from build123d import *

# Parameters (mm, degrees)
SKETCH1_W           = 50
SKETCH1_H           = 50
SKETCH1_R           = 8
BOSS_EXTRUDE1_DEPTH = 1.5
SKETCH4_R           = 1.5
BOSS_EXTRUDE2_DEPTH = 2
BOSS_EXTRUDE3_START = -1.5
SKETCH5_R           = 2.6
SKETCH5_R_2         = 8
BOSS_EXTRUDE3_DEPTH = 1.5
FILLET1_R           = 5
SKETCH6_R           = 5
SKETCH6_R_2         = 2.6
BOSS_EXTRUDE4_DEPTH = 10


with BuildPart() as part:
    # Sketch1 → Boss-Extrude1 (new body)
    with BuildSketch(Plane(origin=(0, 0, 0), x_dir=(1, 0, 0), z_dir=(0, 1, 0))):
        Rectangle(SKETCH1_W, SKETCH1_H)
        with Locations(Location((0, 0, 0), (0, 0, 270))):
            Circle(SKETCH1_R, mode=Mode.SUBTRACT)
    extrude(amount=BOSS_EXTRUDE1_DEPTH)

    # Sketch4 → Boss-Extrude2 (add)
    with BuildSketch(Plane(origin=(0, 1.5, 0), x_dir=(1, 0, 0), z_dir=(0, 1, 0))):
        with Locations(Location((-23, 23, 0), (0, 0, 90))):
            Circle(SKETCH4_R)
        with Locations(Location((-17, 17, 0), (0, 0, 90))):
            Circle(SKETCH4_R)
        with Locations(Location((17, 17, 0), (0, 0, 90))):
            Circle(SKETCH4_R)
        with Locations(Location((23, 23, 0), (0, 0, 90))):
            Circle(SKETCH4_R)
        with Locations(Location((-17, -17, 0), (0, 0, 90))):
            Circle(SKETCH4_R)
        with Locations(Location((-23, -23, 0), (0, 0, 90))):
            Circle(SKETCH4_R)
        with Locations(Location((17, -17, 0), (0, 0, 90))):
            Circle(SKETCH4_R)
        with Locations(Location((23, -23, 0), (0, 0, 90))):
            Circle(SKETCH4_R)
    extrude(amount=BOSS_EXTRUDE2_DEPTH)

    # Sketch5 → Boss-Extrude3 (add)
    with BuildSketch(Plane(origin=(0, 1.5, 0), x_dir=(1, 0, 0), z_dir=(0, 1, 0)).offset(BOSS_EXTRUDE3_START)):
        Polygon((-42.426406871, -35.355339059), (-25, -17.928932188), (-25, 17.928932188), (-42.426406871, 35.355339059), (-45.961940777, 38.890872965), (-38.890872965, 45.961940777), (-35.355339059, 42.426406871), (-17.928932188, 25), (17.928932188, 25), (35.355339059, 42.426406871), (38.890872965, 45.961940777), (45.961940777, 38.890872965), (42.426406871, 35.355339059), (25, 17.928932188), (25, -17.928932188), (42.426406871, -35.355339059), (45.961940777, -38.890872965), (38.890872965, -45.961940777), (35.355339059, -42.426406871), (17.928932188, -25), (-17.928932188, -25), (-35.355339059, -42.426406871), (-38.890872965, -45.961940777), (-45.961940777, -38.890872965), align=None)
        with Locations(Location((-38.890872965, -38.890872965, 0), (0, 0, 270))):
            Circle(SKETCH5_R, mode=Mode.SUBTRACT)
        with Locations(Location((38.890872965, 38.890872965, 0), (0, 0, 270))):
            Circle(SKETCH5_R, mode=Mode.SUBTRACT)
        with Locations(Location((38.890872965, -38.890872965, 0), (0, 0, 90))):
            Circle(SKETCH5_R, mode=Mode.SUBTRACT)
        with Locations(Location((-38.890872965, 38.890872965, 0), (0, 0, 90))):
            Circle(SKETCH5_R, mode=Mode.SUBTRACT)
        with Locations(Location((0, 0, 0), (0, 0, 270))):
            Circle(SKETCH5_R_2, mode=Mode.SUBTRACT)
    extrude(amount=BOSS_EXTRUDE3_DEPTH)

    # Fillet1
    fillet1_edges = [part.edges().sort_by_distance(p)[0] for p in [
        (17.928932188, 0.75, 25),
        (38.890872965, 0.75, 45.961940777),
        (45.961940777, 0.75, 38.890872965),
        (25, 0.75, 17.928932188),
        (25, 0.75, -17.928932188),
        (45.961940777, 0.75, -38.890872965),
        (38.890872965, 0.75, -45.961940777),
        (17.928932188, 0.75, -25),
        (-17.928932188, 0.75, -25),
        (-38.890872965, 0.75, -45.961940777),
        (-45.961940777, 0.75, -38.890872965),
        (-25, 0.75, -17.928932188),
        (-25, 0.75, 17.928932188),
        (-45.961940777, 0.75, 38.890872965),
        (-38.890872965, 0.75, 45.961940777),
        (-17.928932188, 0.75, 25),
    ]]
    fillet(fillet1_edges, radius=FILLET1_R - 0.0001)  # a hair under: the kernel refuses the full size

    # Sketch6 → Boss-Extrude4 (add)
    # profile 1 of 4: a face of its own
    with BuildSketch(Plane(origin=(0, 1.5, 0), x_dir=(1, 0, 0), z_dir=(0, 1, 0))):
        with Locations(Location((-38.890872965, -38.890872965, 0), (0, 0, 270))):
            Circle(SKETCH6_R)
        with Locations(Location((-38.890872965, -38.890872965, 0), (0, 0, 270))):
            Circle(SKETCH6_R_2, mode=Mode.SUBTRACT)
    # profile 2 of 4: a face of its own
    with BuildSketch(Plane(origin=(0, 1.5, 0), x_dir=(1, 0, 0), z_dir=(0, 1, 0))):
        with Locations(Location((-38.890872965, 38.890872965, 0), (0, 0, 270))):
            Circle(SKETCH6_R)
        with Locations(Location((-38.890872965, 38.890872965, 0), (0, 0, 270))):
            Circle(SKETCH6_R_2, mode=Mode.SUBTRACT)
    # profile 3 of 4: a face of its own
    with BuildSketch(Plane(origin=(0, 1.5, 0), x_dir=(1, 0, 0), z_dir=(0, 1, 0))):
        with Locations(Location((38.890872965, 38.890872965, 0), (0, 0, 270))):
            Circle(SKETCH6_R)
        with Locations(Location((38.890872965, 38.890872965, 0), (0, 0, 270))):
            Circle(SKETCH6_R_2, mode=Mode.SUBTRACT)
    # profile 4 of 4: a face of its own
    with BuildSketch(Plane(origin=(0, 1.5, 0), x_dir=(1, 0, 0), z_dir=(0, 1, 0))):
        with Locations(Location((38.890872965, -38.890872965, 0), (0, 0, 270))):
            Circle(SKETCH6_R)
        with Locations(Location((38.890872965, -38.890872965, 0), (0, 0, 270))):
            Circle(SKETCH6_R_2, mode=Mode.SUBTRACT)
    extrude(amount=BOSS_EXTRUDE4_DEPTH)


solid = part.part
Design review of the part built by this model. Coordinates are the model's own, in mm. A direction names the side the tool comes from. Round coordinates to 2 decimals unless told otherwise and drop trailing zeros. Order: outer loops, then holes, each group sorted by start corner. A loop starts at its lowest first (then second) coordinate and runs counter-clockwise, first axis right, second up. Notation, with made-up numbers: M 72.25,75 L 83.25,75 A26 cw 83.25,113 Z; hole C 54,45.25 d11. An arc over 180 degrees is marked long. Answer as CSV lines item,"result". Start each with the question number.
1) Add section D-D (x = 17). Give the boundary of the cut face in (y, z).
2) Tool access review of faces 4 (the face through (-34.56, 0.74, -27.49)), 5 (the face through (-41, 11.5, 41)), 6 (the face through (0, 1.5, 9)), 7 (the face through (27.26, 0.74, 34.33)): name each direction out of +Z, -Z, +X, -X, +Y, -Y from which nothing blocks a thin tool from reaching the whole face with its end or side.
3) Add section C-C (z = 28). Give the boundary of the cut face in (x, y), then the cut area to 3 significant figures.
4) Add section B-B (x = 7). Give the boundary of the cut face in (y, z).
5) Add section A-A (y = 5). Give the boundary of the cut face in (x, z), then the cut area to 3 significant figures.
6) Wall thickness on line 1 along X through (y, z) = (0.7, 0); line 2 along X through (y, z) = (8.75, 40); line 3 along Y through (x, z) = (-14.5, 18): over which ranges is each line inside the solid? List them lowest first. Write a range as [from, to].
7) For pin 1 Ø1.2 at (x, y) = (-1, 0.5) entering from +Z; pin 2 Ø2.5 at (x, z) = (17.5, -17) entering from +Y; pin 3 Ø6 at (x, z) = (29, 24.5) entering from +Y; pin 4 Ø4.5 at (x, z) = (38.89, 38.89) entering from +Y, all flat-tipped, find the tip position at first contact; note any pin that passes through.
8) The part is to be moulded in two halves that separate along X. For faces 1 (the face through (-34.33, 0.74, 27.26)), 2 (the face through (-27.26, 0.74, -34.33)), 3 (the face through (23, 3.5, 23)), say which applies: +X half, -X half, draft (parallel to the pull), parting line (faces both ways), or undercut.
Resolved:
1,outline,"M 0,-25.13 L 1.5,-25.13 L 1.5,-18.5 L 3.5,-18.5 L 3.5,-15.5 L 1.5,-15.5 L 1.5,15.5 L 3.5,15.5 L 3.5,18.5 L 1.5,18.5 L 1.5,25.13 L 0,25.13 Z"
2,face 4,"-X, +Y, -Y"
2,face 5,"+Z, -Z, +X, -X, +Y"
2,face 6,"+Y"
2,face 7,"+Z, +Y, -Y"
3,outline,"M -35.07,0 L -20.93,0 L -20.93,1.5 L -35.07,1.5 Z; M 20.93,0 L 35.07,0 L 35.07,1.5 L 20.93,1.5 Z"
3,area,"42.4 mm^2"
4,outline,"M 0,-25 L 1.5,-25 L 1.5,-3.87 L 0,-3.87 Z; M 0,3.87 L 1.5,3.87 L 1.5,25 L 0,25 Z"
5,outline,"C -38.89,-38.89 d10; C -38.89,38.89 d10; C 38.89,-38.89 d10; C 38.89,38.89 d10; hole C -38.89,-38.89 d5.2; hole C -38.89,38.89 d5.2; hole C 38.89,-38.89 d5.2; hole C 38.89,38.89 d5.2"
5,area,"229 mm^2"
6,line 1,"[-25, -8], [8, 25]"
6,line 2,"[-43.77, -41.24], [-36.54, -34.02], [34.02, 36.54], [41.24, 43.77]"
6,line 3,"[0, 1.5]"
7,pin 1,"z = 25"
7,pin 2,"y = 3.5"
7,pin 3,"y = 1.5"
7,pin 4,"through"
8,face 1,"-X half"
8,face 2,"undercut"
8,face 3,"draft"
